```python
from build123d import *

# Parameters (mm, degrees)
F0_W            = 62
F0_H            = 82
F1_DEPTH        = 12
F2_T1_DEPTH     = 72
F4_R            = 25
F5_DEPTH        = 42.5
F5_DEPTH_BACK   = 39.5
F3_W            = 19
F3_H            = 9
F6_DEPTH        = 88
F8_DEPTH        = 25
F10_DEPTH       = 25
F12_D           = 18
F12_DEPTH       = 90
F12_CBORE_D     = 32
F12_CBORE_DEPTH = 9
F12_TIP         = 5.4077455712


# Not quite as in the source:
# - a fillet or chamfer that OpenCascade refuses, or shapes differently, is made with other operations: its cross-section is extruded or revolved along the edge and cut away or added


with BuildPart() as f1:
    # F0 (on Right) → F1 (new body)
    with BuildSketch(Plane.YZ):
        with Locations((0, 1.4735981822)):
            Rectangle(F0_W, F0_H)
    extrude(amount=F1_DEPTH)

    # F2: fillet of radius 12 on 4 edges, made by hand

    # F2_s2 → F2_t1 (cut)
    with BuildSketch(Plane.YZ.offset(-30)):
        with BuildLine():
            add(Edge.make_bspline(
                [(-19, 42.4735981822), (-31, 42.4735981822), (-31, 30.4735981822)],
                knots=[0, 0, 0, 1, 1, 1], degree=2, weights=[1, 1, 1]))
            Line((-31, 30.4735981822), (-31, 42.4735981822))
            Line((-31, 42.4735981822), (-19, 42.4735981822))
        make_face()
        with BuildLine():
            add(Edge.make_bspline(
                [(31, 30.4735981822), (31, 42.4735981822), (19, 42.4735981822)],
                knots=[0, 0, 0, 1, 1, 1], degree=2, weights=[1, 1, 1]))
            Line((19, 42.4735981822), (31, 42.4735981822))
            Line((31, 42.4735981822), (31, 30.4735981822))
        make_face()
        with BuildLine():
            add(Edge.make_bspline(
                [(-31, -27.5264018178), (-31, -39.5264018178), (-19, -39.5264018178)],
                knots=[0, 0, 0, 1, 1, 1], degree=2, weights=[1, 1, 1]))
            Line((-19, -39.5264018178), (-31, -39.5264018178))
            Line((-31, -39.5264018178), (-31, -27.5264018178))
        make_face()
        with BuildLine():
            add(Edge.make_bspline(
                [(31, -27.5264018178), (31, -39.5264018178), (19, -39.5264018178)],
                knots=[0, 0, 0, 1, 1, 1], degree=2, weights=[1, 1, 1]))
            Line((19, -39.5264018178), (31, -39.5264018178))
            Line((31, -39.5264018178), (31, -27.5264018178))
        make_face()
    extrude(amount=F2_T1_DEPTH, mode=Mode.SUBTRACT)



with BuildPart() as f5:
    # F4 (on Front) → F5 (new body, two sides)
    with BuildSketch(Plane.XZ) as f5_sk:
        with Locations((100, 0)):
            Circle(F4_R)
    extrude(amount=F5_DEPTH)
    extrude(f5_sk.sketch, amount=-F5_DEPTH_BACK)


with BuildPart() as f1_1:
    add(f1.part)

    add(f5.part)  # F6 merges F5
    # F3 (on face) → F6 (join)
    with BuildSketch(Plane.YZ.offset(12)):
        Polygon((4.5, 5.9735981822), (4.5, 42.4735981822), (-4.5, 42.4735981822), (-4.5, 5.9735981822), (-4.5, -3.0264018178), (-4.5, -39.5264018178), (4.5, -39.5264018178), (4.5, -3.0264018178), (23.5, -3.0264018178), (23.5, 5.9735981822), align=None)
        with Locations((-14, 1.4735981822)):
            Rectangle(F3_W, F3_H)
    extrude(amount=F6_DEPTH)

    # F7 (on face) → F8 (cut)
    with BuildSketch(Plane.XZ.offset(4.5)):
        Polygon((100, 42.4735981822), (12, 42.4735981822), (100, 25), align=None)
    extrude(amount=-F8_DEPTH, mode=Mode.SUBTRACT)

    # F9 (on face) → F10 (cut)
    with BuildSketch(Plane.XZ.offset(4.5)):
        Polygon((100, -39.5264018178), (100, -25), (12, -39.5264018178), align=None)
    extrude(amount=-F10_DEPTH, mode=Mode.SUBTRACT)

    # F12
    with Locations(Plane.XZ.offset(42.5)):
        with Locations((100, 0)):
            CounterBoreHole(F12_D / 2, F12_CBORE_D / 2, F12_CBORE_DEPTH, depth=F12_DEPTH)
            with Locations((0, 0, -(F12_DEPTH + F12_TIP / 2))):  # 118° drill point
                Cone(0, F12_D / 2, F12_TIP, mode=Mode.SUBTRACT)


solid = f1_1.part
```
Source: CAD feature listing. Evaluate the final solid. Frame: model axes, mm. A direction names the side the tool comes from. Coordinates: 2 decimals unless noted, no trailing zeros. Write each loop counter-clockwise with the first axis right and the second up, starting at its lowest first coordinate (ties: lowest second). Pieces come first, ordered by that corner, then holes. Notation, with made-up numbers: (18, 56.25) - (77, 56.25) arc R31 cw to (77, 93.25) - close; hole circle Ø11 at (13.5, -14). An arc over 180 degrees is marked (long way). Answer as a JSON object with one key per item and string values.
Q1. Material intervals for line 1 (Z direction, x = 100, y = -36); line 2 (Z direction, x = 100, y = 15.5); line 3 (Y direction, x = 73, z = -23), sorted ascending. Write a range as [from, to].
Ans:
{"line 1": "z = [-25, -16], [16, 25]", "line 2": "z = [-25, -9], [9, 25]", "line 3": "y = [-4.5, 4.5]"}
Q2. Section query A-A, the plane z = 0. Output: boundary loops of the cut face in (x, y).
Ans:
{"outline": "(0, -31) - (12, -31) - (12, -23.5) - (75, -23.5) - (75, -42.5) - (84, -42.5) - (84, -33.5) - (91, -33.5) - (91, 39.5) - (75, 39.5) - (75, 23.5) - (12, 23.5) - (12, 31) - (0, 31) - close; (109, -33.5) - (116, -33.5) - (116, -42.5) - (125, -42.5) - (125, 39.5) - (109, 39.5) - close"}
Q3. Set-up query: faces 5 (the flat face through (43, -14, -3.026)), 6 (the cylindrical face through (123.09, -2.07, -9.58)), 7 (the flat face through (6, 31, 1)). Return all of +Z, -Z, +X, -X, +Y, -Y with unobstructed straight access to the full face (end or side cutting, diameter ignored); none if empty.
Ans:
{"face 5": "-Z, -Y", "face 6": "none", "face 7": "+Z, -Z, -X, +Y"}
Q4. Section query C-C, the plane x = 64.5. Output: boundary loops of the cut face in (y, z).
Ans:
{"outline": "(-23.5, -3.03) - (-4.5, -3.03) - (-4.5, -30.86) - (4.5, -30.86) - (4.5, -3.03) - (23.5, -3.03) - (23.5, 5.97) - (4.5, 5.97) - (4.5, 32.05) - (-4.5, 32.05) - (-4.5, 5.97) - (-23.5, 5.97) - close"}
Q5. Section query D-D, the plane z = 11. Output: boundary loops of the cut face in (x, y).
Ans:
{"outline": "(0, -31) - (12, -31) - (12, -4.5) - (77.55, -4.5) - (77.55, -42.5) - (88.38, -42.5) - (88.38, -33.5) - (111.62, -33.5) - (111.62, -42.5) - (122.45, -42.5) - (122.45, 39.5) - (77.55, 39.5) - (77.55, 4.5) - (12, 4.5) - (12, 31) - (0, 31) - close"}
Q6. Section query B-B, the plane y = -10.5. Output: boundary loops of the cut face in (x, z).
Ans:
{"outline": "(0, -39.53) - (12, -39.53) - (12, -3.03) - (75.18, -3.03) arc R25 ccw (long way) to (75.72, 5.97) - (12, 5.97) - (12, 42.47) - (0, 42.47) - close; hole circle Ø18 at (100, 0)"}
Q7. Draft query along Z for faces 1 (the flat face through (99.6, -42.5, -16.3)), 2 (the flat face through (107, -33.5, -7)), 3 (the cylindrical face through (87.303, -38.063, -9.736)), 4 (the flat face through (43, 14, -3.026)). Return one class per face: released by +Z, released by -Z, zero draft, split by the parting line, or undercut.
Ans:
{"face 1": "zero draft", "face 2": "undercut", "face 3": "undercut", "face 4": "released by -Z"}
Q8. First-contact query: pin 1 Ø10 at (x, y) = (106, 22) entering from -Z; pin 2 Ø15 at (x, y) = (48, 9.5) entering from +Z; pin 3 Ø6 at (x, z) = (6, -3) entering from +Y. Flat tips, straight axial feed; report the tip coordinate or a pass-through.
Ans:
{"pin 1": "stops at z = -24.98", "pin 2": "stops at z = 36.44", "pin 3": "stops at y = 31"}
